For this review, take the finished solid that the model builds, in its own axes (mm). A direction names the side the tool comes from. Round coordinates to 2 decimals unless told otherwise and drop trailing zeros. Write each loop counter-clockwise with the first axis right and the second up, starting at its lowest first coordinate (ties: lowest second). Pieces come first, ordered by that corner, then holes. Notation, with made-up numbers: (-5.5, 40) -> (5.5, 40) arc R16 ccw to (5.5, 50) -> close; hole circle Ø11 at (40.25, 35.5). An arc over 180 degrees is marked (long way). Write each question's results on one line, items separated by ' | '. Start each with the question number.
Item 1: To check wall thickness, follow line 1 along X through (y, z) = (2.5, 45); line 2 along Y through (x, z) = (-2.5, 35). State the ranges of each line that lie inside material, in increasing order.
Item 2: Tool access review of faces 4 (the cylindrical face through (12.45, -12.46, 40.11)), 5 (the cylindrical face through (-14.878, -14.858, 39.425)): name each direction out of +Z, -Z, +X, -X, +Y, -Y from which nothing blocks a thin tool from reaching the whole face with its end or side.
Item 3: Clearance check with flat-ended pins moving along their axes: pin 1 (12 mm diameter, centred on x = 8, y = 7.5, fed in from -Z); pin 2 (8 mm diameter, centred on x = 4.5, z = 8.5, fed in from +Y); pin 3 (6 mm diameter, centred on x = 12, z = 22, fed in from -Y). State where each tip first meets the part, or that it passes through.
Item 4: Add section B-B (z = 46). State the section outline as (x, y) points, plus the area to 3 significant figures.
Item 5: The part is to be moulded in two halves that separate along Y. For faces 1 (the cylindrical face through (-14.858, 14.878, 25.097)), 2 (the flat face through (15.24, 3, 31)), 3 (the flat face through (0, 12.827, 29)), say which applies: +Y half, -Y half, draft (parallel to the pull), parting line (faces both ways), or undercut.
Item 6: Add section A-A (x = -6). State the section outline as (y, z) points, plus the area to 3 significant figures.
Item 7: Add section C-C (x = 10.5). State the section outline as (y, z) points, plus the area to 3 significant figures.
from build123d import *

# Parameters (mm, degrees)
BOSS_EXTRUDE1_DEPTH = 50.8
SKETCH3_R           = 19.05
CUT_EXTRUDE1_DEPTH  = 65.557986338


with BuildPart() as part:
    # Sketch2 → Boss-Extrude1 (new body)
    with BuildSketch(Plane.XY):
        with BuildLine():
            Line((-13.97, -15.24), (13.97, -15.24))
            ThreePointArc((13.97, -15.24), (14.868025612, -14.868025612), (15.24, -13.97))
            Line((15.24, -13.97), (15.24, 13.97))
            ThreePointArc((15.24, 13.97), (14.868025612, 14.868025612), (13.97, 15.24))
            Line((13.97, 15.24), (-13.97, 15.24))
            ThreePointArc((-13.97, 15.24), (-14.868025612, 14.868025612), (-15.24, 13.97))
            Line((-15.24, 13.97), (-15.24, -13.97))
            ThreePointArc((-15.24, -13.97), (-14.868025612, -14.868025612), (-13.97, -15.24))
        make_face()
        with BuildLine():
            Line((-11.557, -12.827), (11.557, -12.827))
            ThreePointArc((11.557, -12.827), (12.455025612, -12.455025612), (12.827, -11.557))
            Line((12.827, -11.557), (12.827, 11.557))
            ThreePointArc((12.827, 11.557), (12.455025612, 12.455025612), (11.557, 12.827))
            Line((11.557, 12.827), (-11.557, 12.827))
            ThreePointArc((-11.557, 12.827), (-12.455025612, 12.455025612), (-12.827, 11.557))
            Line((-12.827, 11.557), (-12.827, -11.557))
            ThreePointArc((-12.827, -11.557), (-12.455025612, -12.455025612), (-11.557, -12.827))
        make_face(mode=Mode.SUBTRACT)
    extrude(amount=BOSS_EXTRUDE1_DEPTH)

    # Sketch3 → Cut-Extrude1 (cut, through all)
    with BuildSketch(Plane(origin=(0, 7.62, -7.62), x_dir=(-1, 0, 0), z_dir=(0, 0.7071067811865464, -0.7071067811865488))):
        with Locations((0, -1.251307345)):
            Circle(SKETCH3_R)
    extrude(amount=-CUT_EXTRUDE1_DEPTH, mode=Mode.SUBTRACT)


solid = part.part
Responses:
1) line 1: x = -15.24 to -12.83, 12.83 to 15.24 | line 2: y = 12.83 to 15.24
2) face 4: +Z, -Z | face 5: +Z, -Z, -X, -Y
3) pin 1: stops at z = 7.09 | pin 2: stops at y = 15.24 | pin 3: stops at y = -7.96
4) outline: (-15.24, -13.97) arc R1.27 ccw to (-13.97, -15.24) -> (13.97, -15.24) arc R1.27 ccw to (15.24, -13.97) -> (15.24, 13.97) arc R1.27 ccw to (13.97, 15.24) -> (-13.97, 15.24) arc R1.27 ccw to (-15.24, 13.97) -> close; hole (-12.83, -11.56) arc R1.27 ccw to (-11.56, -12.83) -> (11.56, -12.83) arc R1.27 ccw to (12.83, -11.56) -> (12.83, 11.56) arc R1.27 ccw to (11.56, 12.83) -> (-11.56, 12.83) arc R1.27 ccw to (-12.83, 11.56) -> close | area: 271 mm^2
5) face 1: +Y half | face 2: draft | face 3: undercut
6) outline: (-15.24, 39.04) -> (-12.83, 36.63) -> (-12.83, 50.8) -> (-15.24, 50.8) -> close; (12.83, 10.97) -> (15.24, 8.56) -> (15.24, 50.8) -> (12.83, 50.8) -> close | area: 130 mm^2
7) outline: (-15.24, 35.95) -> (-12.83, 33.54) -> (-12.83, 50.8) -> (-15.24, 50.8) -> close; (12.83, 7.88) -> (15.24, 5.47) -> (15.24, 50.8) -> (12.83, 50.8) -> close | area: 145 mm^2
